Here's how the part is built. I have some questions about the finished solid (model axes, mm). A direction names the side the tool comes from. Coordinates: 2 decimals unless noted, no trailing zeros. Write each loop counter-clockwise with the first axis right and the second up, starting at its lowest first coordinate (ties: lowest second). Pieces come first, ordered by that corner, then holes. Notation, with made-up numbers: (15.5, -20) - (24.5, -20) arc R26 ccw to (24.5, -2) - close; hole circle Ø8 at (59, -33.5). An arc over 180 degrees is marked (long way). Answer in a Markdown table with one row per item. Add a question column.
Item 1: Imagine slicing it at D-D (z = 1). Please give me the cut outline in (x, y), plus the area to 3 significant figures.
Item 2: We'd pull the mould along X, two halves only. Please class faces 3 (the face through (9, 6.35, 3)), 4 (the face through (0, 3, 6)), 5 (the face through (37.4, 20, 6.3)): +X half, -X half, draft (parallel to the pull), parting line (faces both ways), or undercut.
Item 3: Imagine slicing it at C-C (y = 15). Please give me the cut outline in (x, z).
Item 4: Which directions (+Z, -Z, +X, -X, +Y, -Y) give clear straight access to the entire face, cutting with the end or side of a thin tool? Please do faces 1 (the face through (41, 6.35, 5)), 2 (the face through (25, 0, 6)).
Item 5: I'm going to push flat-ended pins straight in: pin 1 (5 mm diameter, centred on x = 19, z = 2, fed in from -Y); pin 2 (2 mm diameter, centred on y = 17, z = 8.5, fed in from +X); pin 3 (1 mm diameter, centred on y = 9.5, z = 7, fed in from -X); pin 4 (2 mm diameter, centred on x = 16, z = 10.5, fed in from +Y). Where does each tip first touch, or does it pass through?
Item 6: If I drill on probe 1 along Z at (x, y) = (44.45, 4); probe 2 along X at (y, z) = (4.25, 6.35); probe 3 along Y at (x, z) = (5, 10), over which ranges is the centre line in solid material (lowest first)? Write a range as from..to.
Item 7: Imagine slicing it at A-A (z = 6.35). Please give me the cut outline in (x, y).
Item 8: Imagine slicing it at B-B (x = 6.35). Please give me the cut outline in (y, z).
Autodesk Inventor part; units mm, degrees
ref_plane "YZ Plane" through (0, 0, 0) normal (1, 0, 0) x (0, 1, 0)
ref_plane "XZ Plane" through (0, 0, 0) normal (0, 1, 0) x (-1, 0, 0)
ref_plane "XY Plane" through (0, 0, 0) normal (0, 0, 1) x (1, 0, 0)
sketch "Sketch1" plane through (0, 0, 0) normal (0, 0, 1) x (1, 0, 0)
  line L0 (0, 0) -> (50.8, 0)
  arc A0 (37.6547, 6.35) -> (13.1453, 6.35) centre (25.4, 15) ccw
  circle A1 centre (25.4, 15) radius 13
  line L1 (0, 0) -> (0, 6.35)
  line L2 (0, 6.35) -> (13.1453, 6.35)
  line L3 (50.8, 0) -> (50.8, 6.35)
  line L4 (50.8, 6.35) -> (37.6547, 6.35)
  dimension "d0" = 50.8
  dimension "d1" = 30
  dimension "d2" = 26
  dimension "d3" = 6.35
  dimension "d4" = 6.35
  dimension "d5" = 25.4
extrude "Plate1" add sketch "Sketch1" along normal blind 12.7
sketch "Sketch2" plane through (37.6547, 6.35, 0) normal (0, 1, 0) x (1, 0, 0)
  line L0 (0, -12.7) -> (13.1453, -12.7)
  line L1 (13.1453, 0) -> (13.1453, -12.7)
  circle A0 centre (6.7953, -6.35) radius 3.3782
  circle A1 centre (-31.3047, -6.35) radius 3.3782
  line L2 (-37.6547, 0) -> (-37.6547, -12.7)
  line L3 (-24.5094, 0) -> (-37.6547, 0)
  dimension "d7" = 6.7564
  dimension "d8" = 6.7564
  dimension "d9" = 6.35
  dimension "d10" = 6.35
  dimension "d12" = 6.35
  dimension "d13" = 6.35
extrude "Cut1" cut sketch "Sketch2" against normal blind 12.7
equation "\"d14\" = Thickness"
equation "\"BendRadius\" = Thickness"
equation "\"BendReliefWidth\" = Thickness"
equation "\"BendReliefDepth\" = 0.5 * Thickness"
equation "\"CornerReliefSize\" = 4 * Thickness"
equation "\"MinimumRemnant\" = 2 * Thickness"
equation "\"TransitionRadius\" = BendRadius"
equation "\"JacobiRadiusSize\" = BendRadius"
equation "\"GapSize\" = Thickness"
equation "\"d6\" = BendRadius"
properties part number "Pillow block for arm bearing" material "Aluminum 6061"
Here are the results:
| question | item | result |
|---|---|---|
| 1 | outline | (0, 0) - (50.8, 0) - (50.8, 6.35) - (37.65, 6.35) arc R15 ccw (long way) to (13.15, 6.35) - (0, 6.35) - close; hole circle Ø26 at (25.4, 15) |
| 1 | area | 389 mm2 |
| 2 | face 3 | draft |
| 2 | face 4 | -X half |
| 2 | face 5 | undercut |
| 3 | outline | (10.4, 0) - (12.4, 0) - (12.4, 12.7) - (10.4, 12.7) - close; (38.4, 0) - (40.4, 0) - (40.4, 12.7) - (38.4, 12.7) - close |
| 4 | face 1 | +Z, -Z, +X |
| 4 | face 2 | +Z, -Z, +X, -X, -Y |
| 5 | pin 1 | stops at y = 0 |
| 5 | pin 2 | stops at x = 40.37 |
| 5 | pin 3 | stops at x = 11.26 |
| 5 | pin 4 | stops at y = 27.43 |
| 6 | probe 1 | z = 0..2.97, 9.73..12.7 |
| 6 | probe 2 | x = 0..2.97, 9.73..18.09, 32.71..41.07, 47.83..50.8 |
| 6 | probe 3 | y = 0..6.35 |
| 7 | outline | (0, 0) - (2.97, 0) - (2.97, 6.35) - (0, 6.35) - close; (9.73, 0) - (41.07, 0) - (41.07, 6.35) - (37.65, 6.35) arc R15 ccw (long way) to (13.15, 6.35) - (9.73, 6.35) - close; (47.83, 0) - (50.8, 0) - (50.8, 6.35) - (47.83, 6.35) - close; hole circle Ø26 at (25.4, 15) |
| 8 | outline | (0, 0) - (6.35, 0) - (6.35, 2.97) - (0, 2.97) - close; (0, 9.73) - (6.35, 9.73) - (6.35, 12.7) - (0, 12.7) - close |
